Check sheet for the modelled part. Datum: model origin and axes. Units: mm. A direction names the side the tool comes from. Coordinates: 2 decimals unless noted, no trailing zeros. Loops run counter-clockwise (first coordinate to the right, second up) from the corner with the lowest first, then second, coordinate; pieces in that order, holes last. Notation, with made-up numbers: M -30.75,-39 L -6.75,-39 A4 ccw -6.75,-33 Z; hole C 35.5,72.25 d5. An arc over 180 degrees is marked long. Use CSV: the item, a comma, the result in double quotes. Start each with the question number.
(1) Section check B-B on x = 0. Record the cut outline in (y, z), and give its area (3 significant figures).
(2) Go/stop test with flat-tipped pins: pin 1 Ø6 at (x, y) = (-41, 25.5) entering from -Z; pin 2 Ø1.9 at (x, y) = (55.92, 29.97) entering from -Z. Record where each tip stops, or that it passes through.
(3) Set-up check for faces 1 (the flat face through (-63, 0, -16)), 2 (the cylindrical face through (15.09, 15.15, 2.03)), 3 (the cylindrical face through (52.804, -26.934, -18.907)): record each of +Z, -Z, +X, -X, +Y, -Y from which the full face is reachable in a straight line by a thin tool's end or side.
(4) Section check D-D on z = -29. Record the cut outline in (x, y).
(5) Scan lines: line 1 (Y direction, x = 46.5, z = -16); line 2 (X direction, y = -10, z = -19); line 3 (X direction, y = -29.5, z = -33). Record each from-to range of solid material in increasing order.
(6) Section check C-C on z = -6. Record the cut outline in (x, y).
(7) Draft check along Y on faces 4 (the flat face through (-49.719, 0, 2)), 5 (the flat face through (63, 0, -16)), 6 (the flat face through (1, 37.25, -16)). Enter one of: pulls with the +Y half, pulls with the -Y half, needs draft (parallel to the pull), parting line crosses it, or undercut.
(8) Section check A-A on y = -4.5. Record the cut outline in (x, z), and give its area (3 significant figures).
from build123d import *

# Parameters (mm, degrees)
SKETCH_1_W          = 106
SKETCH_1_H          = 54.5
EXTRUDE_1_DEPTH     = 4
SKETCH_2_R          = 2.8
CUT_EXTRUDE_1_DEPTH = 4
SKETCH_3_W          = 103.45800924
SKETCH_3_H          = 52.422924748
EXTRUDE_2_DEPTH     = 41
CUT_EXTRUDE_2_DEPTH = 36.7
EXTRUDE_START       = 36.7
EXTRUDE_3_DEPTH     = 36.7
SKETCH_7_R          = 1.6
CUT_EXTRUDE_3_DEPTH = 20


with BuildPart() as part:
    # Эскиз1 → Бобышка-Вытянуть1 (new body)
    with BuildSketch(Plane.XY):
        Rectangle(SKETCH_1_W, SKETCH_1_H)
    extrude(amount=EXTRUDE_1_DEPTH)

    # Эскиз2 → Вырез-Вытянуть1 (cut)
    with BuildSketch(Plane.XY.offset(4)):
        with Locations((0, -15.15)):
            Circle(SKETCH_2_R)
        with BuildLine():
            Line((-49.719324036, 10.805), (-49.719324036, -10.805))
            ThreePointArc((-49.719324036, -10.805), (-38.819324036, -15.15), (-27.919324036, -10.805))
            Line((-27.919324036, -10.805), (-27.919324036, 10.805))
            ThreePointArc((-27.919324036, 10.805), (-38.819324036, 15.15), (-49.719324036, 10.805))
        make_face()
        with BuildLine():
            Line((-25.819324036, 10.805), (-25.819324036, -10.805))
            ThreePointArc((-25.819324036, -10.805), (-14.919324036, -15.15), (-4.019324036, -10.805))
            Line((-4.019324036, -10.805), (-4.019324036, 10.805))
            ThreePointArc((-4.019324036, 10.805), (-14.919324036, 15.15), (-25.819324036, 10.805))
        make_face()
        with BuildLine():
            Line((4.019324036, 10.805), (4.019324036, -10.805))
            ThreePointArc((4.019324036, -10.805), (14.919324036, -15.15), (25.819324036, -10.805))
            Line((25.819324036, -10.805), (25.819324036, 10.805))
            ThreePointArc((25.819324036, 10.805), (14.919324036, 15.15), (4.019324036, 10.805))
        make_face()
        with BuildLine():
            Line((27.919324036, 10.805), (27.919324036, -10.805))
            ThreePointArc((27.919324036, -10.805), (38.819324036, -15.15), (49.719324036, -10.805))
            Line((49.719324036, -10.805), (49.719324036, 10.805))
            ThreePointArc((49.719324036, 10.805), (38.819324036, 15.15), (27.919324036, 10.805))
        make_face()
    extrude(amount=-CUT_EXTRUDE_1_DEPTH, mode=Mode.SUBTRACT)

    # Эскиз3 → Бобышка-Вытянуть2 (add)
    with BuildSketch(Plane.XY.offset(4)):
        with BuildLine():
            Line((63, -24.419804811), (63, 24.419804811))
            ThreePointArc((63, 24.419804811), (58.922335459, 33.172335459), (50.169804811, 37.25))
            Line((50.169804811, 37.25), (-50.169804811, 37.25))
            ThreePointArc((-50.169804811, 37.25), (-58.922335459, 33.172335459), (-63, 24.419804811))
            Line((-63, 24.419804811), (-63, -24.419804811))
            ThreePointArc((-63, -24.419804811), (-58.922335459, -33.172335459), (-50.169804811, -37.25))
            Line((-50.169804811, -37.25), (50.169804811, -37.25))
            ThreePointArc((50.169804811, -37.25), (58.922335459, -33.172335459), (63, -24.419804811))
        make_face()
        Rectangle(SKETCH_3_W, SKETCH_3_H, mode=Mode.SUBTRACT)
    extrude(amount=-EXTRUDE_2_DEPTH)

    # Эскиз5 → Вырез-Вытянуть2 (cut)
    with BuildSketch(Plane(origin=(0, 0, -37), x_dir=(-1, 0, 0), z_dir=(0, 0, -1))):
        with BuildLine():
            Line((-58, 24.179579232), (-58, -24.179579232))
            ThreePointArc((-58, -24.179579232), (-55.386801553, -29.636801553), (-49.929579232, -32.25))
            Line((-49.929579232, -32.25), (49.929579232, -32.25))
            ThreePointArc((49.929579232, -32.25), (55.386801553, -29.636801553), (58, -24.179579232))
            Line((58, -24.179579232), (58, 24.179579232))
            ThreePointArc((58, 24.179579232), (55.386801553, 29.636801553), (49.929579232, 32.25))
            Line((49.929579232, 32.25), (-49.929579232, 32.25))
            ThreePointArc((-49.929579232, 32.25), (-55.386801553, 29.636801553), (-58, 24.179579232))
        make_face()
    extrude(amount=-CUT_EXTRUDE_2_DEPTH, mode=Mode.SUBTRACT)

    # Эскиз6 → Бобышка-Вытянуть3 (add)
    with BuildSketch(Plane(origin=(0, 0, -0.3), x_dir=(-1, 0, 0), z_dir=(0, 0, -1)).offset(EXTRUDE_START)):
        with BuildLine():
            ThreePointArc((-49.929579232, 32.25), (-52.743515709, 26.993515709), (-58, 24.179579232))
            ThreePointArc((-58, 24.179579232), (-55.386801553, 29.636801553), (-49.929579232, 32.25))
        make_face()
        with BuildLine():
            ThreePointArc((49.929579232, 32.25), (55.386801553, 29.636801553), (58, 24.179579232))
            ThreePointArc((58, 24.179579232), (52.743515709, 26.993515709), (49.929579232, 32.25))
        make_face()
        with BuildLine():
            ThreePointArc((49.929579232, -32.25), (52.743515709, -26.993515709), (58, -24.179579232))
            ThreePointArc((58, -24.179579232), (55.386801553, -29.636801553), (49.929579232, -32.25))
        make_face()
        with BuildLine():
            ThreePointArc((-49.929579232, -32.25), (-55.386801553, -29.636801553), (-58, -24.179579232))
            ThreePointArc((-58, -24.179579232), (-52.743515709, -26.993515709), (-49.929579232, -32.25))
        make_face()
    extrude(amount=-EXTRUDE_3_DEPTH)

    # Эскиз7 → Вырез-Вытянуть3 (cut)
    with BuildSketch(Plane(origin=(0, 0, -37), x_dir=(-1, 0, 0), z_dir=(0, 0, -1))):
        with Locations((-55.91502671, 29.970875188)):
            Circle(SKETCH_7_R)
        with Locations(Location((55.91502671, 29.970875188, 0), (0, 0, 180))):
            Circle(SKETCH_7_R)
        with Locations((55.91502671, -29.970875188)):
            Circle(SKETCH_7_R)
        with Locations(Location((-55.91502671, -29.970875188, 0), (0, 0, 180))):
            Circle(SKETCH_7_R)
    extrude(amount=-CUT_EXTRUDE_3_DEPTH, mode=Mode.SUBTRACT)


solid = part.part
Outcome:
1,outline,"M -37.25,-37 L -32.25,-37 L -32.25,-0.3 L -26.21,-0.3 L -26.21,0 L -17.95,0 L -17.95,4 L -37.25,4 Z; M -12.35,0 L 26.21,0 L 26.21,-0.3 L 32.25,-0.3 L 32.25,-37 L 37.25,-37 L 37.25,4 L -12.35,4 Z"
1,area,"649 mm²"
2,pin 1,"stops at z = -0.3"
2,pin 2,"stops at z = -17"
3,face 1,"+Z, -Z, -X, +Y, -Y"
3,face 2,"+Z, -Z"
3,face 3,"-Z"
4,outline,"M -63,-24.42 A14.1 ccw -50.17,-37.25 L 50.17,-37.25 A14.1 ccw 63,-24.42 L 63,24.42 A14.1 ccw 50.17,37.25 L -50.17,37.25 A14.1 ccw -63,24.42 Z; hole M -58,-24.18 A10.29 cw -49.93,-32.25 L 49.93,-32.25 A10.29 cw 58,-24.18 L 58,24.18 A10.29 cw 49.93,32.25 L -49.93,32.25 A10.29 cw -58,24.18 Z; hole C -55.92,-29.97 d3.2; hole C -55.92,29.97 d3.2; hole C 55.92,-29.97 d3.2; hole C 55.92,29.97 d3.2"
5,line 1,"y = -37.25 to -32.25, 32.25 to 37.25"
5,line 2,"x = -63 to -58, 58 to 63"
5,line 3,"x = -61.57 to -57.44, -54.39 to -50.9, 50.9 to 54.39, 57.44 to 61.57"
6,outline,"M -63,-24.42 A14.1 ccw -50.17,-37.25 L 50.17,-37.25 A14.1 ccw 63,-24.42 L 63,24.42 A14.1 ccw 50.17,37.25 L -50.17,37.25 A14.1 ccw -63,24.42 Z; hole M -58,-24.18 A10.29 cw -49.93,-32.25 L 49.93,-32.25 A10.29 cw 58,-24.18 L 58,24.18 A10.29 cw 49.93,32.25 L -49.93,32.25 A10.29 cw -58,24.18 Z"
7,face 4,"undercut"
7,face 5,"needs draft"
7,face 6,"pulls with the +Y half"
8,outline,"M -63,-37 L -58,-37 L -58,-0.3 L -51.73,-0.3 L -51.73,0 L -49.72,0 L -49.72,4 L -63,4 Z; M -27.92,0 L -25.82,0 L -25.82,4 L -27.92,4 Z; M -4.02,0 L 4.02,0 L 4.02,4 L -4.02,4 Z; M 25.82,0 L 27.92,0 L 27.92,4 L 25.82,4 Z; M 49.72,0 L 51.73,0 L 51.73,-0.3 L 58,-0.3 L 58,-37 L 63,-37 L 63,4 L 49.72,4 Z"
8,area,"529 mm²"
